```python
from build123d import *

# Parameters (mm, degrees)
SKETCH3_W         = 0.79
SKETCH3_H         = 3.1
SKETCH4_W         = 0.395
SKETCH4_H         = 0.395
CIRPATTERN1_COUNT = 2
CIRPATTERN1_ANGLE = 90


with BuildPart() as part:
    # BodySke → Base-Revolve (revolve)
    with BuildSketch(Plane.XY):
        Polygon((0, 0), (0, 2.75), (0.45, 2.75), (1.7, 1.5), (20, 1.5), (20, 0), align=None)
    revolve(axis=Axis((-6.35, 0, 0), (1, 0, 0)))

    # Sketch3 → Cross section 0
    with BuildSketch(Plane.ZY):
        Rectangle(SKETCH3_W, SKETCH3_H)
    # Sketch4 → Cross section 1
    with BuildSketch(Plane.ZY.offset(-2.08)):
        Rectangle(SKETCH4_W, SKETCH4_H)
    cross = loft(mode=Mode.SUBTRACT)

    # CirPattern1: Cross ×2 about axis
    cirpattern1_axis = Axis((0, 0, 0), (1, 0, 0))
    for i in range(1, CIRPATTERN1_COUNT):
        add(cross.rotate(cirpattern1_axis, i * CIRPATTERN1_ANGLE / (CIRPATTERN1_COUNT - 1)), mode=Mode.SUBTRACT)


solid = part.part
```
Can you work these out from the model? Positions are in its coordinate system, mm. A direction names the side the tool comes from. Round coordinates to 2 decimals unless told otherwise and drop trailing zeros. Order: outer loops, then holes, each group sorted by start corner. A loop starts at its lowest first (then second) coordinate and runs counter-clockwise, first axis right, second up. Notation, with made-up numbers: (31, -29) -> (83, -29) arc R30 ccw to (83, 2) -> close; hole circle Ø5 at (61.5, 15). An arc over 180 degrees is marked (long way). Return JSON: item names as keys, results as strings. Group by question number.
1. Will these pins go through, and if not, where does the flat tip stop? pin 1 (1 mm diameter, centred on x = 3.5, z = 1.5, fed in from -Y); pin 2 (1.5 mm diameter, centred on x = 5, z = -1, fed in from -Y); pin 3 (1.5 mm diameter, centred on x = 3, z = -1.5, fed in from -Y).
2. Which directions (+Z, -Z, +X, -X, +Y, -Y) give clear straight access to the entire face, cutting with the end or side of a thin tool? Please do faces 1 (the face through (0, -1, -1)), 2 (the face through (10.98, -1.5, 0.07)).
3. I need wall thicknesses on line 1 (Z direction, x = 16.25, y = -0.05); line 2 (X direction, y = -1.2, z = -1.2); line 3 (X direction, y = 2.2, z = 1.15). Which ranges of each line are inside material? Lowest first, please. Write a range as [from, to].
4. If we section it at A-A, the plane x = 15.5: Write out the boundary of the cut face in (y, z).
Output values:
{
 "1": {"pin 1": "y = -1.12", "pin 2": "y = -1.48", "pin 3": "y = -1.3"},
 "2": {"face 1": "+Z, -Z, -X, +Y, -Y", "face 2": "+X"},
 "3": {"line 1": "[-1.5, 1.5]", "line 2": "[0, 1.5]", "line 3": "[0, 0.72]"},
 "4": {"outline": "circle Ø3 at (0, 0)"}
}
